```python
from build123d import *

# Parameters (mm, degrees)
SKETCH_R  = 2.1
PAD_DEPTH = 250
FILLET_R  = 1.5


with BuildPart() as part:
    # Sketch → Pad (new body, symmetric)
    with BuildSketch(Plane.XZ):
        Polygon((-10, 10), (-3.1, 10), (-3.1, 8.2), (-6, 8.2), (-6, 7.06066), (-2.83934, 3.9), (2.83934, 3.9), (6, 7.06066), (6, 8.2), (3.1, 8.2), (3.1, 10), (16.9, 10), (16.9, 8.2), (14, 8.2), (14, 7.06066), (17.16066, 3.9), (22.83934, 3.9), (26, 7.06066), (26, 8.2), (23.1, 8.2), (23.1, 10), (36.9, 10), (36.9, 8.2), (34, 8.2), (34, 7.06066), (37.16066, 3.9), (42.83934, 3.9), (46, 7.06066), (46, 8.2), (43.1, 8.2), (43.1, 10), (50, 10), (50, 3.1), (48.2, 3.1), (48.2, 6), (47.06066, 6), (43.9, 2.83934), (43.9, -2.83934), (47.06066, -6), (48.2, -6), (48.2, -3.1), (50, -3.1), (50, -10), (43.1, -10), (43.1, -8.2), (46, -8.2), (46, -7.06066), (42.83934, -3.9), (37.16066, -3.9), (34, -7.06066), (34, -8.2), (36.9, -8.2), (36.9, -10), (23.1, -10), (23.1, -8.2), (26, -8.2), (26, -7.06066), (22.83934, -3.9), (17.16066, -3.9), (14, -7.06066), (14, -8.2), (16.9, -8.2), (16.9, -10), (3.1, -10), (3.1, -8.2), (6, -8.2), (6, -7.06066), (2.83934, -3.9), (-2.83934, -3.9), (-6, -7.06066), (-6, -8.2), (-3.1, -8.2), (-3.1, -10), (-10, -10), (-10, -3.1), (-8.2, -3.1), (-8.2, -6), (-7.06066, -6), (-3.9, -2.83934), (-3.9, 2.83934), (-7.06066, 6), (-8.2, 6), (-8.2, 3.1), (-10, 3.1), align=None)
        Circle(SKETCH_R, mode=Mode.SUBTRACT)
        with Locations((20, 0)):
            Circle(SKETCH_R, mode=Mode.SUBTRACT)
        with Locations((39.9, 0)):
            Circle(SKETCH_R, mode=Mode.SUBTRACT)
        Polygon((7.8, -6.53934), (4.1, -2.83934), (4.1, 2.83934), (7.8, 6.53934), (7.8, 8.2), (12.2, 8.2), (12.2, 6.53934), (15.9, 2.83934), (15.9, -2.83934), (12.2, -6.53934), (12.2, -8.2), (7.8, -8.2), align=None, mode=Mode.SUBTRACT)
        Polygon((27.8, 8.2), (27.8, 6.53934), (24.1, 2.83934), (24.1, -2.83934), (27.8, -6.53934), (27.8, -8.2), (32.2, -8.2), (32.2, -6.53934), (35.9, -2.83934), (35.9, 2.83934), (32.2, 6.53934), (32.2, 8.2), align=None, mode=Mode.SUBTRACT)
    extrude(amount=PAD_DEPTH, both=True)

    # Fillet
    fillet_edges = [part.edges().sort_by_distance(p)[0] for p in [
        (-10, 0, 10),
        (50, 0, 10),
        (-10, 0, -10),
        (50, 0, -10),
    ]]
    fillet(fillet_edges, radius=FILLET_R)


with BuildPart() as part_1:
    # Body placement: moved
    add(part.part.moved(Location((-30, 0, 0))))


solid = part_1.part
```
Check sheet for the modelled part. Datum: model origin and axes. Units: mm. Coordinates: 2 decimals unless noted, no trailing zeros. One line per question, with ' | ' between items.
Item 1: Gauge pin test, flat ends, axial feed: P1, Ø5, axis at x = -30.5, y = 75.5, coming from the +Z side; P2, Ø1.7, axis at x = 10.5, y = 92, coming from the +Z side; P3, Ø4.5, axis at y = -19, z = 0.5, coming from the -X side. Record the tip position at first contact, or that the pin passes through.
Determined:
P1: stops at z = 4.06 | P2: stops at z = 3.9 | P3: stops at x = -33.9
Item 2: Thickness scan on line 1 (X direction, y = -215, z = -7.5); line 2 (X direction, y = 143, z = -7); line 3 (Z direction, x = -19.5, y = 223.5). Record the ranges inside material, lowest first. Write a range as [from, to].
Determined:
line 1: x = [-40, -36], [-24, -22.2], [-17.8, -16], [-4, -2.2], [2.2, 4], [16, 20] | line 2: x = [-40, -35.94], [-24.06, -22.2], [-17.8, -15.94], [-4.06, -2.2], [2.2, 4.06], [15.94, 20] | line 3: z = [-10, -8.2], [8.2, 10]
Item 3: Sectioned sample at A-A on y = -7.5. Give the number of separate pieces and of enclosed holes in the cut face, plus the area to 3 significant figures.
Determined:
separate pieces: 1 | enclosed holes: 5 | area: 451 mm2
